from build123d import *

# Parameters (mm, degrees)
SKETCH1_R           = 1.5
SKETCH1_R_2         = 6.9
BOSS_EXTRUDE1_DEPTH = 9
BOSS_EXTRUDE2_DEPTH = 9


with BuildPart() as part:
    # Sketch1 → Boss-Extrude1 (new body)
    with BuildSketch(Plane(origin=(0, 0, 0), x_dir=(1, 0, 0), z_dir=(0, 1, 0))):
        with BuildLine():
            Line((-11.652723828, -50.570490945), (4.846773171, -50.570490945))
            Line((4.846773171, -50.570490945), (8.637408256, -56.047889168))
            ThreePointArc((8.637408256, -56.047889168), (11.767276172, -66.070490945), (14.897144088, -56.047889168))
            Line((14.897144088, -56.047889168), (18.687779173, -50.570490945))
            Line((18.687779173, -50.570490945), (35.187276172, -50.570490945))
            Line((35.187276172, -50.570490945), (40.187276172, -55.570490945))
            Line((40.187276172, -55.570490945), (40.187276172, -87.300490945))
            Line((40.187276172, -87.300490945), (35.187276172, -92.300490945))
            Line((35.187276172, -92.300490945), (-11.652723828, -92.300490945))
            Line((-11.652723828, -92.300490945), (-16.652723828, -87.300490945))
            Line((-16.652723828, -87.300490945), (-16.652723828, -55.570490945))
            Line((-16.652723828, -55.570490945), (-11.652723828, -50.570490945))
        make_face()
        with Locations(Location((11.767276172, -73.315490945, 0), (0, 0, 270))):
            Circle(SKETCH1_R, mode=Mode.SUBTRACT)
        with Locations(Location((11.767276172, -83.315490945, 0), (0, 0, 270))):
            Circle(SKETCH1_R, mode=Mode.SUBTRACT)
        with Locations(Location((-4.752723828, -80.400490945, 0), (0, 0, 270))):
            Circle(SKETCH1_R_2, mode=Mode.SUBTRACT)
        with Locations(Location((28.287276172, -80.400490945, 0), (0, 0, 270))):
            Circle(SKETCH1_R_2, mode=Mode.SUBTRACT)
    extrude(amount=BOSS_EXTRUDE1_DEPTH)

    # Sketch2 → Boss-Extrude2 (add)
    with BuildSketch(Plane(origin=(0, 9, 0), x_dir=(1, 0, 0), z_dir=(0, 1, 0))):
        Polygon((26.099816941, -36.988069685), (20.899816941, -36.988069685), (18.687779173, -50.570490945), (35.187276172, -50.570490945), (40.187276172, -55.570490945), (40.187276172, -60.936255598), (47.560429658, -50.288069685), (47.560429658, -36.988069685), (42.490429658, -36.988069685), (42.490429658, -46.788069685), (26.099816941, -46.788069685), align=None)
        Polygon((-18.955877314, -36.988069685), (-24.025877314, -36.988069685), (-24.025877314, -50.288069685), (-16.652723828, -60.936255598), (-16.652723828, -55.570490945), (-11.652723828, -50.570490945), (4.846773171, -50.570490945), (2.634735403, -36.988069685), (-2.565264597, -36.988069685), (-2.565264597, -46.788069685), (-18.955877314, -46.788069685), align=None)
    extrude(amount=-BOSS_EXTRUDE2_DEPTH)


solid = part.part
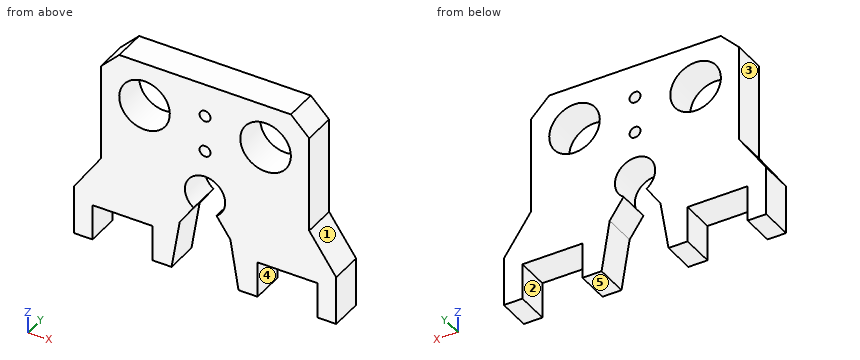
Model file for the job. Use its own axes, mm. Face numbers are marked on the shaded views. A direction names the side the tool comes from. Give positions to 0.01 mm unless a question says otherwise; leave off trailing zeros. Loops run counter-clockwise (first coordinate to the right, second up) from the corner with the lowest first, then second, coordinate; pieces in that order, holes last.
Item 1: Slice it at B-B (z = 80). Write the cut outline in (x, y), plus the area to 3 significant figures.
Check values:
outline: (-16.65, 0) - (-11.64, 0) - (-11.64, 9) - (-16.65, 9) - close; (2.14, 0) - (21.4, 0) - (21.4, 9) - (2.14, 9) - close; (35.18, 0) - (40.19, 0) - (40.19, 9) - (35.18, 9) - close
area: 264 mm2
Item 2: Slice it at A-A (x = 12.5). Write the cut outline in (y, z).
Check values:
outline: (0, 66.02) - (9, 66.02) - (9, 72.01) - (0, 72.01) - close; (0, 74.62) - (9, 74.62) - (9, 82.01) - (0, 82.01) - close; (0, 84.62) - (9, 84.62) - (9, 92.3) - (0, 92.3) - close
Item 3: Drop flat-ended pins along their axis: P1, Ø1, axis at y = 2.5, z = 54, coming from the +X side; P2, Ø5, axis at y = 4.5, z = 72.5, coming from the +X side; P3, Ø5, axis at y = 5.5, z = 58.5, coming from the -X side. Give the stop position or say it passes through.
Check values:
P1: stops at x = 45.34
P2: stops at x = 40.19
P3: stops at x = -20.07
Item 4: Mould opens along X. For the marked faces 3, 4 and 5 say: +X half, -X half, draft (parallel to the pull), parting line (faces both ways), or undercut.
Check values:
face 3: -X half
face 4: undercut
face 5: draft
Item 5: Drill centre lines: line 1 along X through (y, z) = (6.25, 80); line 2 along X through (y, z) = (6, 43.5); line 3 along X through (y, z) = (2.75, 85.5). Where is each one in solid material? Low to high.
Check values:
line 1: x = -16.65 to -11.64, 2.14 to 21.4, 35.18 to 40.19
line 2: x = -24.03 to -18.96, -2.57 to 3.7, 19.84 to 26.1, 42.49 to 47.56
line 3: x = -16.65 to -9.4, -0.1 to 23.64, 32.94 to 40.19
Item 6: Which spindle directions (+Z, -Z, +X, -X, +Y, -Y) get a long thin tool onto all of the face, cutting with end or side? Do the marked faces 1 and 2. Say none if no direction does.
Check values:
face 1: +Z, +X, +Y, -Y
face 2: -Z, +Y, -Y
Item 7: Slice it at D-D (y = 1). Write the cut outline in (x, z).
Check values:
outline: (-24.03, 36.99) - (-18.96, 36.99) - (-18.96, 46.79) - (-2.57, 46.79) - (-2.57, 36.99) - (2.63, 36.99) - (4.85, 50.57) - (8.64, 56.05) arc R5.5 cw (long way) to (14.9, 56.05) - (18.69, 50.57) - (20.9, 36.99) - (26.1, 36.99) - (26.1, 46.79) - (42.49, 46.79) - (42.49, 36.99) - (47.56, 36.99) - (47.56, 50.29) - (40.19, 60.94) - (40.19, 87.3) - (35.19, 92.3) - (-11.65, 92.3) - (-16.65, 87.3) - (-16.65, 60.94) - (-24.03, 50.29) - close; hole circle Ø13.8 at (-4.75, 80.4); hole circle Ø3 at (11.77, 73.32); hole circle Ø3 at (11.77, 83.32); hole circle Ø13.8 at (28.29, 80.4)
Item 8: Slice it at C-C (x = -3.5). Write the cut outline in (y, z), plus the area to 3 significant figures.
Check values:
outline: (0, 46.79) - (9, 46.79) - (9, 73.62) - (0, 73.62) - close; (0, 87.19) - (9, 87.19) - (9, 92.3) - (0, 92.3) - close
area: 287 mm2
